Input: part model. Units: mm. Frame: model coordinates. Coordinates: 2 decimals unless noted, no trailing zeros. Write each loop counter-clockwise with the first axis right and the second up, starting at its lowest first coordinate (ties: lowest second). Pieces come first, ordered by that corner, then holes. Notation, with made-up numbers: (58.5, 82.5) - (101.5, 82.5) arc R24 ccw to (101.5, 107.5) - close; hole circle Ø9 at (89.25, -8.5). An arc over 180 degrees is marked (long way). Use CSV: the item, a comma, the result in double quotes.
```python
from build123d import *

# Parameters (mm, degrees)
SKETCH1_W           = 9
SKETCH1_H           = 110
BOSS_EXTRUDE2_DEPTH = 7
SKETCH4_R           = 1.5
CUT_EXTRUDE2_DEPTH  = 10
SKETCH6_R           = 1.5
CUT_EXTRUDE4_DEPTH  = 10
FILLET1_R           = 1.5
FILLET2_R           = 1.5


with BuildPart() as part:
    # Sketch1 → Boss-Extrude2 (new body)
    with BuildSketch(Plane.XY):
        with Locations((3.95483871, 54.062211982)):
            Rectangle(SKETCH1_W, SKETCH1_H)
    extrude(amount=BOSS_EXTRUDE2_DEPTH)

    # Sketch4 → Cut-Extrude2 (cut, through all)
    with BuildSketch(Plane(origin=(8.45483871, 0, 0), x_dir=(0, 0, -1), z_dir=(1, 0, 0))):
        with Locations((-3.5, 2.062211982)):
            Circle(SKETCH4_R)
    extrude(amount=-CUT_EXTRUDE2_DEPTH, mode=Mode.SUBTRACT)

    # Sketch6 → Cut-Extrude4 (cut, through all)
    with BuildSketch(Plane(origin=(8.45483871, 0, 0), x_dir=(0, 0, -1), z_dir=(1, 0, 0))):
        with Locations((-3.5, 106.062211982)):
            Circle(SKETCH6_R)
    extrude(amount=-CUT_EXTRUDE4_DEPTH, mode=Mode.SUBTRACT)

    # Fillet1
    fillet1_edges = [part.edges().sort_by_distance(p)[0] for p in [
        (3.95483871, 109.062211982, 7),
        (3.95483871, 109.062211982, 0),
    ]]
    fillet(fillet1_edges, radius=FILLET1_R)

    # Fillet2
    fillet2_edges = [part.edges().sort_by_distance(p)[0] for p in [
        (3.95483871, -0.937788018, 7),
        (3.95483871, -0.937788018, 0),
    ]]
    fillet(fillet2_edges, radius=FILLET2_R)


solid = part.part
```
(1) Cut plane A-A on z = 3.5. Return loops of the section in (x, y), and give its area (3 significant figures).
Check values:
outline,"(-0.55, -0.94) - (8.45, -0.94) - (8.45, 0.56) - (-0.55, 0.56) - close; (-0.55, 3.56) - (8.45, 3.56) - (8.45, 104.56) - (-0.55, 104.56) - close; (-0.55, 107.56) - (8.45, 107.56) - (8.45, 109.06) - (-0.55, 109.06) - close"
area,"936 mm^2"
(2) Cut plane B-B on x = 3.5. Return loops of the section in (y, z), and give its area (3 significant figures).
Check values:
outline,"(-0.94, 1.5) arc R1.5 ccw to (0.56, 0) - (107.56, 0) arc R1.5 ccw to (109.06, 1.5) - (109.06, 5.5) arc R1.5 ccw to (107.56, 7) - (0.56, 7) arc R1.5 ccw to (-0.94, 5.5) - close; hole circle Ø3 at (2.06, 3.5); hole circle Ø3 at (106.06, 3.5)"
area,"754 mm^2"
(3) Ray query, probe 1 along Y at (x, z) = (5.5, 3.5); probe 2 along Y at (x, z) = (7.5, 3.75); probe 3 along Y at (x, z) = (6.5, 6.75). Return the intervals inside material, ascending. Write a range as from..to.
Check values:
probe 1,"-0.94..0.56, 3.56..104.56, 107.56..109.06"
probe 2,"-0.94..0.58, 3.54..104.58, 107.54..109.06"
probe 3,"-0.27..108.39"
(4) Draft query along Y for faces 1 (the flat face through (8.455, 53, 3)), 2 (the flat face through (4, -0.938, 3)), 3 (the cylindrical face through (4.018, 1.488, 2.114)), 4 (the cylindrical face through (4.018, 107.327, 2.694)). Return one class per face: pulls with the +Y half, pulls with the -Y half, needs draft (parallel to the pull), parting line crosses it, or undercut.
Check values:
face 1,"needs draft"
face 2,"pulls with the -Y half"
face 3,"undercut"
face 4,"undercut"
